Geometry: final body of the model. Coordinates: model frame, mm. A direction names the side the tool comes from. Give positions to 0.01 mm unless a question says otherwise; leave off trailing zeros. Loops run counter-clockwise (first coordinate to the right, second up) from the corner with the lowest first, then second, coordinate; pieces in that order, holes last. Notation, with made-up numbers: (74.25, -39) -> (91.25, -39) arc R29 cw to (91.25, -7) -> close; hole circle Ø5 at (65, 74). An arc over 180 degrees is marked (long way). Answer in a Markdown table with one row per item. Add a question column.
from build123d import *

# Parameters (mm, degrees)
BOSS_EXTRU_1_OUTLINE_R   = 2
BOSS_EXTRU_1_OUTLINE_W   = 10
BOSS_EXTRU_1_OUTLINE_H   = 2
BOSS_EXTRU_1_OUTLINE_W_2 = 2
BOSS_EXTRU_1_OUTLINE_H_2 = 10
BOSS_EXTRU_1_DEPTH       = 5
BOSS_EXTRU_2_DEPTH       = 5
CONG_1_R                 = 5


with BuildPart() as part:
    # Boss.-Extru.1: read off the stored shape, not the designer's step
    # Boss.-Extru.1 outline → Boss.-Extru.1 (new body)
    with BuildSketch(Plane.XY):
        with BuildLine():
            ThreePointArc((60, 0), (-15.529142706, 57.955549577), (-51.961524227, -30))
            Line((-51.961524227, -30), (60, -30))
            Line((60, -30), (60, 0))
        make_face()
        with Locations((-30, -20)):
            Circle(BOSS_EXTRU_1_OUTLINE_R, mode=Mode.SUBTRACT)
        with Locations((-50, 0)):
            Rectangle(BOSS_EXTRU_1_OUTLINE_W, BOSS_EXTRU_1_OUTLINE_H, mode=Mode.SUBTRACT)
        Polygon((-53.990778238, 10.535457525), (-44.142700708, 8.798975748), (-44.489997063, 6.829360242), (-54.338074593, 8.565842019), align=None, mode=Mode.SUBTRACT)
        Circle(BOSS_EXTRU_1_OUTLINE_R, mode=Mode.SUBTRACT)
        with Locations((30, -20)):
            Circle(BOSS_EXTRU_1_OUTLINE_R, mode=Mode.SUBTRACT)
        with Locations((50, 0)):
            Rectangle(BOSS_EXTRU_1_OUTLINE_W, BOSS_EXTRU_1_OUTLINE_H, mode=Mode.SUBTRACT)
        Polygon((54.338074593, 8.565842019), (44.489997063, 6.829360242), (44.142700708, 8.798975748), (53.990778238, 10.535457525), align=None, mode=Mode.SUBTRACT)
        Polygon((-51.341074, 19.750800504), (-41.944147792, 16.33059907), (-42.628188079, 14.451213829), (-52.025114287, 17.871415262), align=None, mode=Mode.SUBTRACT)
        Polygon((-47.131397208, 28.366025404), (-38.47114317, 23.366025404), (-39.47114317, 21.633974596), (-48.131397208, 26.633974596), align=None, mode=Mode.SUBTRACT)
        Polygon((-41.489656762, 36.119362976), (-33.829212331, 29.691486879), (-35.11478755, 28.159397993), (-42.775231981, 34.58727409), align=None, mode=Mode.SUBTRACT)
        with BuildLine():
            ThreePointArc((-28, 0), (-30, -2), (-32, 0))
            ThreePointArc((-32, 0), (0, 32), (32, 0))
            ThreePointArc((32, 0), (30, -2), (28, 0))
            ThreePointArc((28, 0), (0, 28), (-28, 0))
        make_face(mode=Mode.SUBTRACT)
        Polygon((-34.58727409, 42.775231981), (-28.159397993, 35.11478755), (-29.691486879, 33.829212331), (-36.119362976, 41.489656762), align=None, mode=Mode.SUBTRACT)
        Polygon((-26.633974596, 48.131397208), (-21.633974596, 39.47114317), (-23.366025404, 38.47114317), (-28.366025404, 47.131397208), align=None, mode=Mode.SUBTRACT)
        Polygon((-17.871415262, 52.025114287), (-14.451213829, 42.628188079), (-16.33059907, 41.944147792), (-19.750800504, 51.341074), align=None, mode=Mode.SUBTRACT)
        Polygon((-8.565842019, 54.338074593), (-6.829360242, 44.489997063), (-8.798975748, 44.142700708), (-10.535457525, 53.990778238), align=None, mode=Mode.SUBTRACT)
        with Locations((0, 50)):
            Rectangle(BOSS_EXTRU_1_OUTLINE_W_2, BOSS_EXTRU_1_OUTLINE_H_2, mode=Mode.SUBTRACT)
        Polygon((48.131397208, 26.633974596), (39.47114317, 21.633974596), (38.47114317, 23.366025404), (47.131397208, 28.366025404), align=None, mode=Mode.SUBTRACT)
        Polygon((52.025114287, 17.871415262), (42.628188079, 14.451213829), (41.944147792, 16.33059907), (51.341074, 19.750800504), align=None, mode=Mode.SUBTRACT)
        Polygon((42.775231981, 34.58727409), (35.11478755, 28.159397993), (33.829212331, 29.691486879), (41.489656762, 36.119362976), align=None, mode=Mode.SUBTRACT)
        Polygon((19.750800504, 51.341074), (16.33059907, 41.944147792), (14.451213829, 42.628188079), (17.871415262, 52.025114287), align=None, mode=Mode.SUBTRACT)
        Polygon((28.366025404, 47.131397208), (23.366025404, 38.47114317), (21.633974596, 39.47114317), (26.633974596, 48.131397208), align=None, mode=Mode.SUBTRACT)
        Polygon((10.535457525, 53.990778238), (8.798975748, 44.142700708), (6.829360242, 44.489997063), (8.565842019, 54.338074593), align=None, mode=Mode.SUBTRACT)
        Polygon((36.119362976, 41.489656762), (29.691486879, 33.829212331), (28.159397993, 35.11478755), (34.58727409, 42.775231981), align=None, mode=Mode.SUBTRACT)
    extrude(amount=BOSS_EXTRU_1_DEPTH)

    # Esquisse2 → Boss.-Extru.2 (add)
    with BuildSketch(Plane.XY.offset(5)):
        Polygon((69, -22), (72, -22), (72, -25), (77, -25), (77, -30), (72, -30), (60, -30), (60, -10), (72, -10), (77, -10), (77, -15), (72, -15), (72, -18), (69, -18), (69, -16.5), (66, -16.5), (66, -18), (62, -18), (62, -22), (66, -22), (66, -23.5), (69, -23.5), align=None)
    extrude(amount=-BOSS_EXTRU_2_DEPTH)

    # Congé1
    cong_1_edges = [part.edges().sort_by_distance(p)[0] for p in [
        (-51.961524227, -30, 2.5),
        (60, -10, 2.5),
    ]]
    fillet(cong_1_edges, radius=CONG_1_R)


solid = part.part
(1) Draft query along X for faces 3 (the flat face through (60, -3, 2)), 4 (the cylindrical face through (-12.545, 58.674, 2.465)), 5 (the flat face through (50, -1, 2)). Return one class per face: +X half, -X half, draft (parallel to the pull), parting line (faces both ways), or undercut.
(2) Pin query (flat end, axial travel): pin 1 Ø6 at (x, y) = (62.5, 10) entering from -Z; pin 2 Ø1.2 at (x, z) = (64.5, 1.5) entering from +Y; pin 3 Ø2.5 at (y, z) = (-3, 3.5) entering from +X; pin 4 Ø3 at (x, z) = (-7, 2) entering from +Y. Return the tip coordinate at first contact, or that it passes through.
(3) Cut plane A-A on y = -20. Return the cut outline in (x, z).
(4) Reachability of faces 1 (the flat face through (-9.655, 48.998, 2.465)), 2 (the flat face through (64, -18, 3)) from +Z, -Z, +X, -X, +Y, -Y: full face, straight path, thin tool, end or side. Return the list, or none.
(5) Material intervals for line 1 along Y through (x, z) = (0, 3.95); line 2 along X through (y, z) = (12, 3.25); line 3 along Y through (x, z) = (-51, 0.5), sorted ascending. Write a range as from..to.
(6) Cut plane B-B on z = 3.55. State how many separate pieces and enclosed holes the cut face has, then the cut area to 3 significant figures.
Answer list:
| question | item | result |
|---|---|---|
| 1 | face 3 | +X half |
| 1 | face 4 | parting line |
| 1 | face 5 | undercut |
| 2 | pin 1 | passes through |
| 2 | pin 2 | stops at y = -9.88 |
| 2 | pin 3 | stops at x = 60 |
| 2 | pin 4 | stops at y = 59.75 |
| 3 | outline | (-56.57, 0) -> (-32, 0) -> (-32, 5) -> (-56.57, 5) -> close; (-28, 0) -> (28, 0) -> (28, 5) -> (-28, 5) -> close; (32, 0) -> (62, 0) -> (62, 5) -> (32, 5) -> close |
| 4 | face 1 | +Z, -Z |
| 4 | face 2 | +Z, -Z, +X |
| 5 | line 1 | y = -30..-2, 2..28, 32..45, 55..60 |
| 5 | line 2 | x = -58.79..-29.66, -25.3..25.3, 29.66..58.79 |
| 5 | line 3 | y = -29.58..-1, 1..7.98, 10.01..17.5, 19.63..31.61 |
| 6 | separate pieces | 1 |
| 6 | enclosed holes | 23 |
| 6 | area | 8,610 mm² |
